Source: CAD feature listing. Evaluate the final solid. Frame: model axes, mm. A direction names the side the tool comes from. Round coordinates to 2 decimals unless told otherwise and drop trailing zeros. Write each loop counter-clockwise with the first axis right and the second up, starting at its lowest first coordinate (ties: lowest second). Pieces come first, ordered by that corner, then holes. Notation, with made-up numbers: (-20, -19.75) -> (20, -19.75) arc R18 ccw to (20, -8.75) -> close; hole circle Ø5 at (13.25, 23). An arc over 180 degrees is marked (long way). Return JSON: item names as keys, results as strings. Group by question number.
from build123d import *

# Parameters (mm, degrees)
EXTRUDE_1_DEPTH     = 26
SKETCH_2_R          = 1
CUT_EXTRUDE_1_DEPTH = 3


with BuildPart() as part:
    # 草图1 → 凸台-拉伸1 (new body)
    with BuildSketch(Plane(origin=(0, 0, 0), x_dir=(1, 0, 0), z_dir=(0, 1, 0))):
        Polygon((-8.5, 0), (8.5, 0), (8.5, -7), (3.517553147, -7), (3.517553147, -5), (1.508639639, -4.25), (3.5, -3.5), (3.5, -3), (-3.5, -3), (-3.5, -3.5), (-1.508639639, -4.25), (-3.517553147, -5), (-3.517553147, -7), (-8.5, -7), align=None)
    extrude(amount=EXTRUDE_1_DEPTH)

    # 草图2 → 切除-拉伸1 (cut)
    with BuildSketch(Plane(origin=(0, 0, 0), x_dir=(-1, 0, 0), z_dir=(0, 0, -1))):
        with Locations((6, 19.5)):
            Circle(SKETCH_2_R)
        with Locations((6, 6.5)):
            Circle(SKETCH_2_R)
        with Locations(Location((-6, 6.5, 0), (0, 0, 180))):
            Circle(SKETCH_2_R)
        with Locations(Location((-6, 19.5, 0), (0, 0, 180))):
            Circle(SKETCH_2_R)
    extrude(amount=-CUT_EXTRUDE_1_DEPTH, mode=Mode.SUBTRACT)


solid = part.part
Item 1: Cut plane D-D on x = -2.5. Output: boundary loops of the cut face in (y, z), and give its area (3 significant figures).
Item 2: First-contact query: pin 1 Ø1 at (x, y) = (-5, 12) entering from -Z; pin 2 Ø3.5 at (x, y) = (1.5, 15) entering from +Z; pin 3 Ø0.6 at (x, y) = (6, 19) entering from -Z. Flat tips, straight axial feed; report the tip coordinate or a pass-through.
Item 3: Cut plane A-A on z = 2.5. Output: boundary loops of the cut face in (x, y), and give its area (3 significant figures).
Item 4: Cut plane B-B on y = 21.5. Output: boundary loops of the cut face in (x, z), and give its area (3 significant figures).
Item 5: Set-up query: faces 1 (the flat face through (8.5, 13, 3)), 2 (the flat face through (0, 13, 0)), 3 (the cylindrical face through (5.783, 20.476, 1.479)), 4 (the flat face through (0, 13, 3)), 5 (the flat face through (-3.518, 13, 6)). Return all of +Z, -Z, +X, -X, +Y, -Y with unobstructed straight access to the full face (end or side cutting, diameter ignored); none if empty.
Item 6: Cut plane C-C on z = 6. Output: boundary loops of the cut face in (x, y), and give its area (3 significant figures).
Item 7: Pull-direction query (X, two-part tool) for faces 6 (the flat face through (6, 6, 3)), 7 (the flat face through (0.1, 0, 2.7)), 8 (the flat face through (-8.5, 13, 4)); classes: +X half, -X half, draft (parallel to the pull), parting line (faces both ways), or undercut.
Item 8: Material intervals for probe 1 along Y at (x, z) = (6, 1.6); probe 2 along X at (y, z) = (15.5, 5.75); probe 3 along Z at (x, y) = (-0.25, 24.75), sorted ascending.
Here are the results:
{
 "1": {"outline": "(0, 0) -> (26, 0) -> (26, 3) -> (0, 3) -> close; (0, 3.88) -> (26, 3.88) -> (26, 4.62) -> (0, 4.62) -> close", "area": "97.3 mm^2"},
 "2": {"pin 1": "stops at z = 0", "pin 2": "stops at z = 4.9", "pin 3": "stops at z = 3"},
 "3": {"outline": "(-8.5, 0) -> (8.5, 0) -> (8.5, 26) -> (-8.5, 26) -> close; hole circle Ø2 at (-6, 6.5); hole circle Ø2 at (-6, 19.5); hole circle Ø2 at (6, 6.5); hole circle Ø2 at (6, 19.5)", "area": "429 mm^2"},
 "4": {"outline": "(-8.5, 0) -> (8.5, 0) -> (8.5, 7) -> (3.52, 7) -> (3.52, 5) -> (1.51, 4.25) -> (3.5, 3.5) -> (3.5, 3) -> (-3.5, 3) -> (-3.5, 3.5) -> (-1.51, 4.25) -> (-3.52, 5) -> (-3.52, 7) -> (-8.5, 7) -> close", "area": "93.9 mm^2"},
 "5": {"face 1": "+Z, -Z, +X, +Y, -Y", "face 2": "-Z, +X, -X, +Y, -Y", "face 3": "-Z", "face 4": "+Y, -Y", "face 5": "+Z, +Y, -Y"},
 "6": {"outline": "(-8.5, 0) -> (-3.52, 0) -> (-3.52, 26) -> (-8.5, 26) -> close; (3.52, 0) -> (8.5, 0) -> (8.5, 26) -> (3.52, 26) -> close", "area": "259 mm^2"},
 "7": {"face 6": "undercut", "face 7": "draft", "face 8": "-X half"},
 "8": {"probe 1": "y = 0 to 5.5, 7.5 to 18.5, 20.5 to 26", "probe 2": "x = -8.5 to -3.52, 3.52 to 8.5", "probe 3": "z = 0 to 3"}
}
